The drawing under review shows one solid part. Ordinate dimensions are in mm from its lowest x, y, z. A direction names the side the tool comes from. Coordinates: 2 decimals unless noted, no trailing zeros. Loops run counter-clockwise (first coordinate to the right, second up) from the corner with the lowest first, then second, coordinate; pieces in that order, holes last. Notation, with made-up numbers: M -29,67 L 5,67 A35 cw 5,100 Z; hole C -33,0.25 d10. An arc over 180 degrees is marked long. Use one line per item in the form item = value.
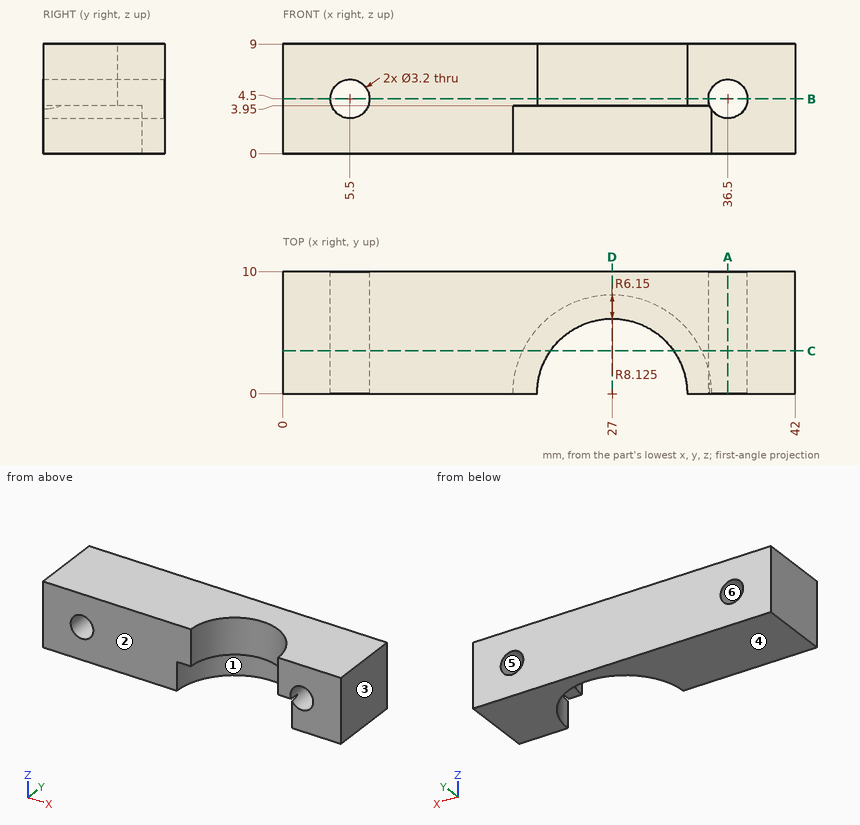
1. Consider section A-A on x = 36.5. Write out the cut boundary in (y, z), plus the area to 3 significant figures.
Computed values:
outline = M 0,0 L 10,0 L 10,2.9 L 0,2.9 Z; M 0,6.1 L 10,6.1 L 10,9 L 0,9 Z
area = 58.0 mm2
2. Wall thickness on line 1 along Z through (x, y) = (36.5, 7.5); line 2 along X through (y, z) = (6.75, 5); line 3 along X through (y, z) = (3, 1.75): over which ranges is each line inside the solid? List them lowest first. Write a range as from..to.
Computed values:
line_1 = 0..2.9, 6.1..9
line_2 = 0..3.98, 7.02..34.98, 38.02..42
line_3 = 0..19.45, 34.55..42
3. Consider section D-D on x = 27. Write out the cut boundary in (y, z) (3 decimals).
Computed values:
outline = M 6.15,3.95 L 8.125,3.95 L 8.125,0 L 10,0 L 10,9 L 6.15,9 Z
4. Tool access review of the marked faces 1 and 2: name each direction out of +Z, -Z, +X, -X, +Y, -Y from which nothing blocks a thin tool from reaching the whole face with its end or side.
Computed values:
face_1 = -Z, -Y
face_2 = +Z, -Z, +X, -X, -Y
5. Consider section B-B on z = 4.5. Write out the cut boundary in (x, y).
Computed values:
outline = M 0,0 L 3.9,0 L 3.9,10 L 0,10 Z; M 7.1,0 L 20.85,0 A6.15 cw 33.15,0 L 34.9,0 L 34.9,10 L 7.1,10 Z; M 38.1,0 L 42,0 L 42,10 L 38.1,10 Z
6. Draft analysis for pull direction X (two halves, no side actions). For the marked faces 3, 4, 5 and 6, state which applies: +X half, -X half, draft (parallel to the pull), parting line (faces both ways), or undercut.
Computed values:
face_3 = +X half
face_4 = draft
face_5 = undercut
face_6 = undercut
7. For pin 1 Ø5 at (y, z) = (6.5, 5) entering from -X; pin 2 Ø1.9 at (x, z) = (5.5, 4.5) entering from -Y; pin 3 Ø4 at (x, z) = (24.5, 2.5) entering from -Y, all flat-tipped, find the tip position at first contact; note any pin that passes through.
Computed values:
pin_1 = 0
pin_2 = through
pin_3 = 4.77
8. Consider section C-C on y = 3.5. Write out the cut boundary in (x, z).
Computed values:
outline = M 0,0 L 19.67,0 L 19.67,3.95 L 21.94,3.95 L 21.94,9 L 0,9 Z; M 32.06,3.95 L 34.33,3.95 L 34.33,0 L 42,0 L 42,9 L 32.06,9 Z; hole C 5.5,4.5 d3.2; hole C 36.5,4.5 d3.2
